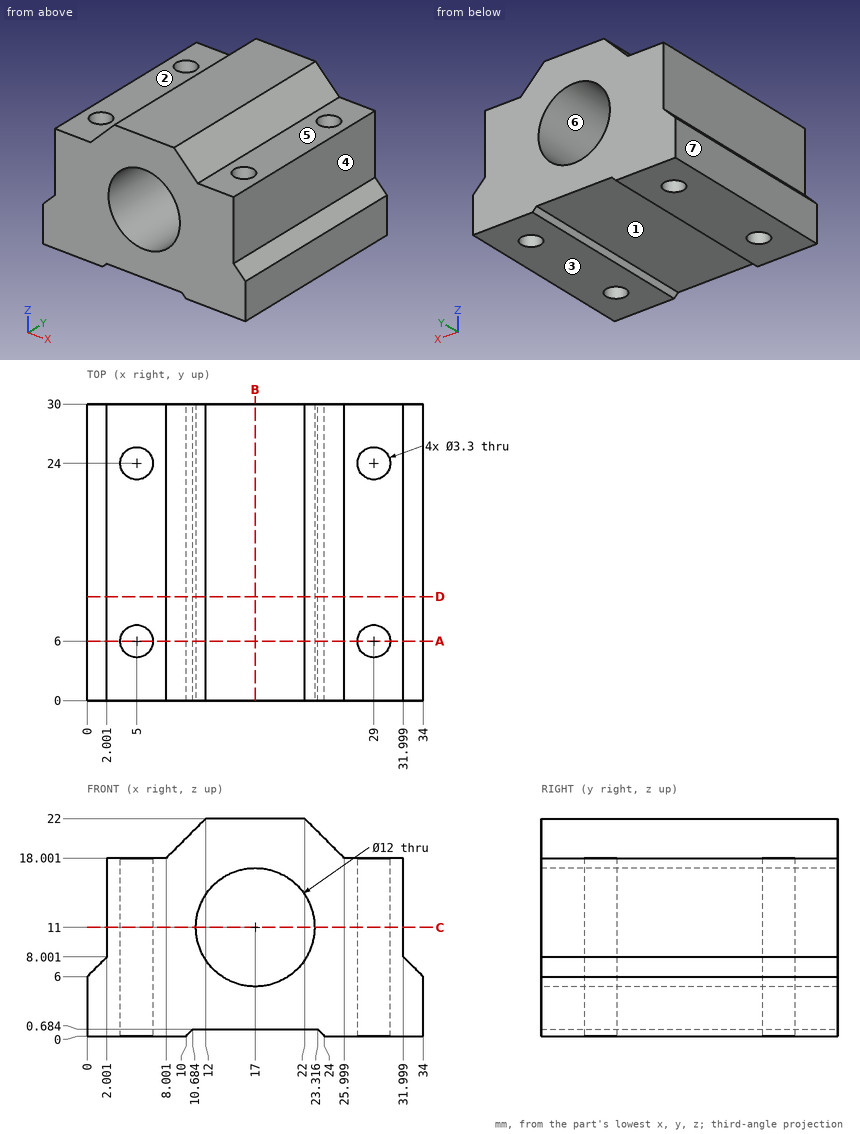
Input: dimensioned drawing with shaded views. Units: mm. Origin: part minimum x, y, z. A direction names the side the tool comes from. Round coordinates to 2 decimals unless told otherwise and drop trailing zeros. Loops run counter-clockwise (first coordinate to the right, second up) from the corner with the lowest first, then second, coordinate; pieces in that order, holes last. Notation, with made-up numbers: (22.5, -34) -> (73.5, -34) arc R15 cw to (73.5, -17) -> close; hole circle Ø8 at (88, -37). An arc over 180 degrees is marked (long way). Answer as a JSON object with one key per item and string values. Group by question number.
Q1. Access query for the marked faces 1, 2, 3 and 4. Directions: +Z, -Z, +X, -X, +Y, -Y. A direction counts if a zero-diameter tool reaches every point of the face in a straight line with its end or side. Return the directions, or none.
Q2. Section query A-A (y = 6). Output: boundary loops of the cut face in (x, z), plus the area to 3 significant figures.
Q3. Contact query for flat-ended pins moving along their axis: P1, Ø2.5, axis at x = 29, y = 6, coming from the +Z side; P2, Ø8, axis at y = 20.5, z = 11, coming from the -X side; P3, Ø4, axis at x = 5, y = 24, coming from the +Z side; P4, Ø6.5, axis at x = 5, y = 22, coming from the +Z side. Output: stop coordinate, or through.
Q4. Mould query, pull axis X, two halves, no side actions, for the marked faces 5, 6 and 7. Classes: pulls with the +X half, pulls with the -X half, needs draft (parallel to the pull), parting line crosses it, or undercut.
Q5. Section query C-C (z = 11). Output: boundary loops of the cut face in (x, y), plus the area to 3 significant figures.
Q6. Section query B-B (x = 17). Output: boundary loops of the cut face in (y, z).
Q7. Ray query, line 1 (Y direction, x = 5, z = 12.25); line 2 (Y direction, x = 28, z = 10.25); line 3 (X direction, y = 10.25, z = 11). Return the intervals inside material, ascending. Write a range as from..to.
Q8. Section query D-D (y = 10.5). Output: boundary loops of the cut face in (x, z), plus the area to 3 significant figures.
Completed:
{
 "1": {"face 1": "-Z, +Y, -Y", "face 2": "+Z, -X, +Y, -Y", "face 3": "-Z, +X, -X, +Y, -Y", "face 4": "+Z, +X, +Y, -Y"},
 "2": {"outline": "(0, 0) -> (3.35, 0) -> (3.35, 18) -> (2, 18) -> (2, 8) -> (0, 6) -> close; (6.65, 0) -> (10, 0) -> (10.68, 0.68) -> (23.32, 0.68) -> (24, 0) -> (27.35, 0) -> (27.35, 18) -> (26, 18) -> (22, 22) -> (12, 22) -> (8, 18) -> (6.65, 18) -> close; (30.65, 0) -> (34, 0) -> (34, 6) -> (32, 8) -> (32, 18) -> (30.65, 18) -> close; hole circle Ø12 at (17, 11)", "area": "383 mm²"},
 "3": {"P1": "through", "P2": "x = 1", "P3": "z = 18", "P4": "z = 18.25"},
 "4": {"face 5": "needs draft", "face 6": "undercut", "face 7": "pulls with the -X half"},
 "5": {"outline": "(2, 0) -> (11, 0) -> (11, 30) -> (2, 30) -> close; (23, 0) -> (32, 0) -> (32, 30) -> (23, 30) -> close; hole circle Ø3.3 at (5, 6); hole circle Ø3.3 at (5, 24); hole circle Ø3.3 at (29, 6); hole circle Ø3.3 at (29, 24)", "area": "506 mm²"},
 "6": {"outline": "(0, 0.68) -> (30, 0.68) -> (30, 5) -> (0, 5) -> close; (0, 17) -> (30, 17) -> (30, 22) -> (0, 22) -> close"},
 "7": {"line 1": "0..4.35, 7.65..22.35, 25.65..30", "line 2": "0..4.69, 7.31..22.69, 25.31..30", "line 3": "2..11, 23..32"},
 "8": {"outline": "(0, 0) -> (10, 0) -> (10.68, 0.68) -> (23.32, 0.68) -> (24, 0) -> (34, 0) -> (34, 6) -> (32, 8) -> (32, 18) -> (26, 18) -> (22, 22) -> (12, 22) -> (8, 18) -> (2, 18) -> (2, 8) -> (0, 6) -> close; hole circle Ø12 at (17, 11)", "area": "502 mm²"}
}
